Geometry check sheet. Reference: the model listing, model coordinates, mm. Face numbers are marked on the shaded views. A direction names the side the tool comes from. Round coordinates to 2 decimals unless told otherwise and drop trailing zeros. Write each loop counter-clockwise with the first axis right and the second up, starting at its lowest first coordinate (ties: lowest second). Pieces come first, ordered by that corner, then holes. Notation, with made-up numbers: M -1,51.5 L 53,51.5 A14 cw 53,69.5 Z; hole C 36,2 d5. An arc over 180 degrees is marked long. Put each result on its own line as item: value. Start each with the question number.
(1) Section check A-A on y = -27. Record the cut outline in (x, z).
(2) Material ranges on probe 1 along Y at (x, z) = (-40, -7.7); probe 2 along Z at (x, y) = (-15.5, 19.5); probe 3 along X at (y, z) = (27, 22.85), recorded low to high.
(3) Mould release check, pull along Z, two halves, no side actions. Record for the marked faces 1, 2 and 3: pulls with the +Z half, pulls with the -Z half, needs draft (parallel to the pull), parting line crosses it, or undercut.
(4) Section check B-B on z = 11. Record the cut outline in (x, y).
(5) Section check C-C on y = -6. Record the cut outline in (x, z), then the cut area to 3 significant figures.
(6) Section check D-D on x = -40. Count the separate pieces of the cut face and the enclosed holes in it, then the cut area to 3 significant figures.
(7) Tool access check on the marked faces 4 and 5. Record the directions out of +Z, -Z, +X, -X, +Y, -Y that give a thin tool (end or side, any length) a straight path to the whole face; none if there is none.
from build123d import *

# Parameters (mm, degrees)
SKETCH1_W           = 78
SKETCH1_H           = 100
SKETCH1_R           = 5
BOSS_EXTRUDE1_DEPTH = 15
FILLET1_R           = 10
SKETCH2_W           = 78
SKETCH2_H           = 7.5
BOSS_EXTRUDE2_DEPTH = 50
SKETCH3_W           = 78
SKETCH3_H           = 1
BOSS_EXTRUDE3_DEPTH = 100
FILLET2_R           = 10
FILLET3_R           = 10
CUT_EXTRUDE1_START  = -100
SKETCH4_R           = 5
CUT_EXTRUDE1_DEPTH  = 100


with BuildPart() as part:
    # Sketch1 → Boss-Extrude1 (new body)
    with BuildSketch(Plane(origin=(0, 0, 0), x_dir=(0, 1, 0), z_dir=(0, 0, 1))):
        with Locations((0, 5)):
            Rectangle(SKETCH1_W, SKETCH1_H)
        with Locations(Location((-27, 40, 0), (0, 0, 270))):
            Circle(SKETCH1_R, mode=Mode.SUBTRACT)
        with Locations(Location((27, 40, 0), (0, 0, 90))):
            Circle(SKETCH1_R, mode=Mode.SUBTRACT)
    extrude(amount=BOSS_EXTRUDE1_DEPTH)

    # Fillet1
    fillet1_edges = [part.edges().sort_by_distance(p)[0] for p in [
        (-55, -39, 7.5),
        (-55, 39, 7.5),
    ]]
    fillet(fillet1_edges, radius=FILLET1_R)

    # Sketch2 → Boss-Extrude2 (add)
    with BuildSketch(Plane.YZ.offset(45)):
        with Locations((0, 18.75)):
            Rectangle(SKETCH2_W, SKETCH2_H)
        with Locations((0, -3.75)):
            Rectangle(SKETCH2_W, SKETCH2_H)
    extrude(amount=-BOSS_EXTRUDE2_DEPTH)

    # Sketch3 → Boss-Extrude3 (add)
    with BuildSketch(Plane.YZ.offset(45)):
        with Locations((0, 23)):
            Rectangle(SKETCH3_W, SKETCH3_H)
        with Locations((0, -8)):
            Rectangle(SKETCH3_W, SKETCH3_H)
    extrude(amount=-BOSS_EXTRUDE3_DEPTH)

    # Fillet2
    fillet2_edges = [part.edges().sort_by_distance(p)[0] for p in [
        (-55, 39, -8),
        (-55, -39, -8),
        (45, 39, 7.5),
        (45, -39, 7.5),
    ]]
    fillet(fillet2_edges, radius=FILLET2_R)

    # Fillet3
    fillet3_edges = [part.edges().sort_by_distance(p)[0] for p in [
        (-55, -39, 23),
        (-55, 39, 23),
    ]]
    fillet(fillet3_edges, radius=FILLET3_R)

    # Sketch4 → Cut-Extrude1 (cut)
    with BuildSketch(Plane.XY.offset(23.5).offset(CUT_EXTRUDE1_START)):
        with Locations(Location((-40, 27, 0), (0, 0, 180))):
            Circle(SKETCH4_R)
        with Locations((-40, -27)):
            Circle(SKETCH4_R)
    extrude(amount=CUT_EXTRUDE1_DEPTH, mode=Mode.SUBTRACT)


solid = part.part
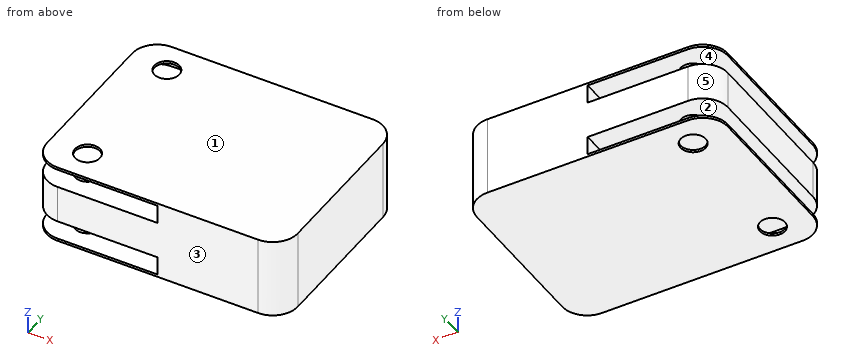
Answers follow:
1. outline: M -55,-8.5 L -45,-8.5 L -45,-7.5 L -55,-7.5 Z; M -55,0 L -45,0 L -45,15 L -55,15 Z; M -55,22.5 L -45,22.5 L -45,23.5 L -55,23.5 Z; M -35,-8.5 L 45,-8.5 L 45,23.5 L -35,23.5 L -35,22.5 L -5,22.5 L -5,15 L -35,15 L -35,0 L -5,0 L -5,-7.5 L -35,-7.5 Z
2. probe 1: y = -39 to -32, -22 to 22, 32 to 39
2. probe 2: z = -8.5 to -7.5, 0 to 15, 22.5 to 23.5
2. probe 3: x = -55 to -45, -35 to 45
3. face 1: pulls with the +Z half
3. face 2: undercut
3. face 3: needs draft
4. outline: M -55,-29 A10 ccw -45,-39 L 35,-39 A10 ccw 45,-29 L 45,29 A10 ccw 35,39 L -45,39 A10 ccw -55,29 Z; hole C -40,-27 d10; hole C -40,27 d10
5. outline: M -55,-8.5 L 45,-8.5 L 45,23.5 L -55,23.5 L -55,22.5 L -5,22.5 L -5,15 L -55,15 L -55,0 L -5,0 L -5,-7.5 L -55,-7.5 Z
5. area: 2,450 mm^2
6. separate pieces: 9
6. enclosed holes: 0
6. area: 986 mm^2
7. face 4: -X, +Y, -Y
7. face 5: +Z, -Z, -X, +Y
